Verification items for the finished model (mm, model axes). A direction names the side the tool comes from. Give positions to 0.01 mm unless a question says otherwise; leave off trailing zeros. Loops run counter-clockwise (first coordinate to the right, second up) from the corner with the lowest first, then second, coordinate; pieces in that order, holes last. Notation, with made-up numbers: (41.5, -32) - (55.5, -32) arc R15 ccw to (55.5, -20) - close; hole circle Ø5 at (48.25, 66.25). An arc over 180 degrees is marked (long way). Answer in a Markdown table with one row per item.
```python
from build123d import *

# Parameters (mm, degrees)
SKETCH_1_W           = 250
SKETCH_1_H           = 250
EXTRUDE_1_DEPTH      = 3
SKETCH_2_W           = 250
SKETCH_2_H           = 250
SKETCH_2_W_2         = 240
SKETCH_2_H_2         = 240
EXTRUDE_2_DEPTH      = 250
SKETCH_3_W           = 3
SKETCH_3_H           = 240
EXTRUDE_3_DEPTH      = 250
SKETCH_8_W           = 200
SKETCH_8_H           = 165
CUT_EXTRUDE_4_DEPTH  = 8
SKETCH_9_W           = 220
SKETCH_9_H           = 185
CUT_EXTRUDE_5_DEPTH  = 3
SKETCH_11_W          = 142
SKETCH_11_H          = 168
CUT_EXTRUDE_6_DEPTH  = 10
SKETCH_12_W          = 162
SKETCH_12_H          = 188
CUT_EXTRUDE_7_DEPTH  = 3
SKETCH_16_W          = 26
SKETCH_16_H          = 18
CUT_EXTRUDE_10_DEPTH = 5
SKETCH_17_W          = 9
SKETCH_17_H          = 11
SKETCH_17_W_2        = 15
SKETCH_17_H_2        = 8
CUT_EXTRUDE_11_DEPTH = 10
SKETCH_21_W          = 28
SKETCH_21_H          = 28
CUT_EXTRUDE_14_DEPTH = 3
SKETCH_22_W          = 50
SKETCH_22_H          = 3
EXTRUDE_4_DEPTH      = 240
SKETCH_24_R          = 4
CUT_EXTRUDE_15_DEPTH = 10
SKETCH_25_W          = 210
SKETCH_25_H          = 132
CUT_EXTRUDE_16_DEPTH = 10
SKETCH_26_R          = 1.25
CUT_EXTRUDE_17_DEPTH = 10
SKETCH_27_R          = 5
CUT_EXTRUDE_18_DEPTH = 10
SKETCH_29_W          = 35
SKETCH_29_H          = 70
CUT_EXTRUDE_19_DEPTH = 10
SKETCH_30_R          = 1.25
CUT_EXTRUDE_20_DEPTH = 3
SKETCH_31_W          = 3
SKETCH_31_H          = 15
EXTRUDE_5_DEPTH      = 3
SKETCH_32_W          = 3
SKETCH_32_H          = 15
EXTRUDE_6_DEPTH      = 3
SKETCH_33_R          = 1.25
CUT_EXTRUDE_21_DEPTH = 7
FILLET_1_R           = 3


with BuildPart() as part:
    # Эскиз1 → Бобышка-Вытянуть1 (new body)
    with BuildSketch(Plane(origin=(0, 0, 0), x_dir=(1, 0, 0), z_dir=(0, 1, 0))):
        Rectangle(SKETCH_1_W, SKETCH_1_H)
    extrude(amount=EXTRUDE_1_DEPTH)

    # Эскиз2 → Бобышка-Вытянуть2 (add)
    with BuildSketch(Plane(origin=(0, 3, 0), x_dir=(1, 0, 0), z_dir=(0, 1, 0))):
        Rectangle(SKETCH_2_W, SKETCH_2_H)
        Rectangle(SKETCH_2_W_2, SKETCH_2_H_2, mode=Mode.SUBTRACT)
    extrude(amount=EXTRUDE_2_DEPTH)

    # Эскиз3 → Бобышка-Вытянуть3 (add)
    with BuildSketch(Plane(origin=(0, 3, 0), x_dir=(1, 0, 0), z_dir=(0, 1, 0))):
        with Locations((-68.5, 0)):
            Rectangle(SKETCH_3_W, SKETCH_3_H)
    extrude(amount=EXTRUDE_3_DEPTH)

    # Эскиз8 → Вырез-Вытянуть4 (cut)
    with BuildSketch(Plane(origin=(125, 0, 0), x_dir=(0, 0, -1), z_dir=(1, 0, 0))):
        with Locations((0, 155.5)):
            Rectangle(SKETCH_8_W, SKETCH_8_H)
    extrude(amount=-CUT_EXTRUDE_4_DEPTH, mode=Mode.SUBTRACT)

    # Эскиз9 → Вырез-Вытянуть5 (cut)
    with BuildSketch(Plane.ZY.offset(-120)):
        with Locations((0, 155.5)):
            Rectangle(SKETCH_9_W, SKETCH_9_H)
    extrude(amount=-CUT_EXTRUDE_5_DEPTH, mode=Mode.SUBTRACT)

    # Эскиз11 → Вырез-Вытянуть6 (cut)
    with BuildSketch(Plane.XY.offset(125)):
        with Locations((29, 154)):
            Rectangle(SKETCH_11_W, SKETCH_11_H)
    extrude(amount=-CUT_EXTRUDE_6_DEPTH, mode=Mode.SUBTRACT)

    # Эскиз12 → Вырез-Вытянуть7 (cut)
    with BuildSketch(Plane(origin=(0, 0, 120), x_dir=(-1, 0, 0), z_dir=(0, 0, -1))):
        with Locations((-29, 154)):
            Rectangle(SKETCH_12_W, SKETCH_12_H)
    extrude(amount=-CUT_EXTRUDE_7_DEPTH, mode=Mode.SUBTRACT)

    # Эскиз16 → Вырез-Вытянуть10 (cut)
    with BuildSketch(Plane.XY.offset(125)):
        with Locations((-95, 128)):
            Rectangle(SKETCH_16_W, SKETCH_16_H)
    extrude(amount=-CUT_EXTRUDE_10_DEPTH, mode=Mode.SUBTRACT)

    # Эскиз17 → Вырез-Вытянуть11 (cut)
    with BuildSketch(Plane.ZY.offset(125)):
        with Locations((105.5, 80.5)):
            Rectangle(SKETCH_17_W, SKETCH_17_H)
        with Locations((73.5, 79)):
            Rectangle(SKETCH_17_W_2, SKETCH_17_H_2)
    extrude(amount=-CUT_EXTRUDE_11_DEPTH, mode=Mode.SUBTRACT)

    # Эскиз21 → Вырез-Вытянуть14 (cut)
    with BuildSketch(Plane(origin=(0, 0, 120), x_dir=(-1, 0, 0), z_dir=(0, 0, -1))):
        with Locations((95, 128)):
            Rectangle(SKETCH_21_W, SKETCH_21_H)
    extrude(amount=-CUT_EXTRUDE_14_DEPTH, mode=Mode.SUBTRACT)

    # Эскиз22 → Бобышка-Вытянуть4 (add)
    with BuildSketch(Plane.XY.offset(-120)):
        with Locations((-95, 71.5)):
            Rectangle(SKETCH_22_W, SKETCH_22_H)
    extrude(amount=EXTRUDE_4_DEPTH)

    # Эскиз24 → Вырез-Вытянуть15 (cut)
    with BuildSketch(Plane(origin=(-67, 0, 0), x_dir=(0, 0, -1), z_dir=(1, 0, 0))):
        with Locations((110, 65)):
            Circle(SKETCH_24_R)
    extrude(amount=-CUT_EXTRUDE_15_DEPTH, mode=Mode.SUBTRACT)

    # Эскиз25 → Вырез-Вытянуть16 (cut)
    with BuildSketch(Plane.ZY.offset(125)):
        with Locations((0, 167)):
            Rectangle(SKETCH_25_W, SKETCH_25_H)
    extrude(amount=-CUT_EXTRUDE_16_DEPTH, mode=Mode.SUBTRACT)

    # Эскиз26 → Вырез-Вытянуть17 (cut)
    with BuildSketch(Plane.ZY.offset(125)):
        with Locations((-110, 238)):
            Circle(SKETCH_26_R)
        with Locations((110, 238)):
            Circle(SKETCH_26_R)
        with Locations((110, 96)):
            Circle(SKETCH_26_R)
        with Locations((-110, 96)):
            Circle(SKETCH_26_R)
    extrude(amount=-CUT_EXTRUDE_17_DEPTH, mode=Mode.SUBTRACT)

    # Эскиз27 → Вырез-Вытянуть18 (cut)
    with BuildSketch(Plane(origin=(0, 73, 0), x_dir=(1, 0, 0), z_dir=(0, 1, 0))):
        with Locations(Location((-95, 10, 0), (0, 0, 270))):
            Circle(SKETCH_27_R)
    extrude(amount=-CUT_EXTRUDE_18_DEPTH, mode=Mode.SUBTRACT)

    # Эскиз29 → Вырез-Вытянуть19 (cut)
    with BuildSketch(Plane(origin=(0, 73, 0), x_dir=(1, 0, 0), z_dir=(0, 1, 0))):
        with Locations((-95, 65)):
            Rectangle(SKETCH_29_W, SKETCH_29_H)
    extrude(amount=-CUT_EXTRUDE_19_DEPTH, mode=Mode.SUBTRACT)

    # Эскиз30 → Вырез-Вытянуть20 (cut)
    with BuildSketch(Plane(origin=(0, 73, 0), x_dir=(1, 0, 0), z_dir=(0, 1, 0))):
        with Locations(Location((-75, 105, 0), (0, 0, 270))):
            Circle(SKETCH_30_R)
        with Locations(Location((-115, 105, 0), (0, 0, 270))):
            Circle(SKETCH_30_R)
        with Locations(Location((-115, 25, 0), (0, 0, 270))):
            Circle(SKETCH_30_R)
        with Locations(Location((-75, 25, 0), (0, 0, 270))):
            Circle(SKETCH_30_R)
    extrude(amount=-CUT_EXTRUDE_20_DEPTH, mode=Mode.SUBTRACT)

    # Эскиз31 → Бобышка-Вытянуть5 (add)
    with BuildSketch(Plane.XY.offset(-120)):
        with Locations((118.5, 245.5)):
            Rectangle(SKETCH_31_W, SKETCH_31_H)
        with Locations((-118.5, 245.5)):
            Rectangle(SKETCH_31_W, SKETCH_31_H)
    extrude(amount=EXTRUDE_5_DEPTH)

    # Эскиз32 → Бобышка-Вытянуть6 (add)
    with BuildSketch(Plane(origin=(0, 0, 120), x_dir=(-1, 0, 0), z_dir=(0, 0, -1))):
        with Locations((-118.5, 245.5)):
            Rectangle(SKETCH_32_W, SKETCH_32_H)
        with Locations((118.5, 245.5)):
            Rectangle(SKETCH_32_W, SKETCH_32_H)
    extrude(amount=EXTRUDE_6_DEPTH)

    # Эскиз33 → Вырез-Вытянуть21 (cut)
    with BuildSketch(Plane(origin=(0, 253, 0), x_dir=(1, 0, 0), z_dir=(0, 1, 0))):
        with Locations(Location((-121, -121, 0), (0, 0, 270))):
            Circle(SKETCH_33_R)
        with Locations(Location((-121, 121, 0), (0, 0, 270))):
            Circle(SKETCH_33_R)
        with Locations(Location((121, 121, 0), (0, 0, 270))):
            Circle(SKETCH_33_R)
        with Locations(Location((121, -121, 0), (0, 0, 270))):
            Circle(SKETCH_33_R)
    extrude(amount=-CUT_EXTRUDE_21_DEPTH, mode=Mode.SUBTRACT)

    # Скругление1
    fillet_1_edges = [part.edges().sort_by_distance(p)[0] for p in [
        (117, 245.5, -117),
        (-117, 245.5, -117),
        (117, 245.5, 117),
        (-117, 245.5, 117),
    ]]
    fillet(fillet_1_edges, radius=FILLET_1_R - 0.0001)  # a hair under: the kernel refuses the full size


solid = part.part
```
Q1. Draft check along X on faces 1 (the face through (-30, 69, 125)), 2 (the face through (-125, 97, 2)), 3 (the face through (-95, 73, 25)). Enter one of: +X half, -X half, draft (parallel to the pull), parting line (faces both ways), or undercut.
Completed:
| item | result |
|---|---|
| face 1 | draft |
| face 2 | -X half |
| face 3 | undercut |
Q2. Thickness scan on line 1 (X direction, y = 71.15, z = -10); line 2 (X direction, y = 249, z = 121); line 3 (Y direction, x = -109.5, z = 62). Record the ranges inside material, lowest first.
Completed:
| item | result |
|---|---|
| line 1 | -125 to -100, -90 to -67, 123 to 125 |
| line 2 | -125 to -122.25, -119.75 to 119.75, 122.25 to 125 |
| line 3 | 0 to 3, 70 to 73 |
Q3. Sectioned sample at C-C (z = -10). Give the number of separate pieces and of enclosed holes in the cut face, and give its area (4 significant figures).
Completed:
| item | result |
|---|---|
| separate pieces | 3 |
| enclosed holes | 0 |
| area | 2,575 mm^2 |
Q4. Tool access check on faces 4 (the face through (-70, 36, 2)), 5 (the face through (-99.88, 71.52, -11.08)), 6 (the face through (-56, 253, -121)). Record the directions out of +Z, -Z, +X, -X, +Y, -Y that give a thin tool (end or side, any length) a straight path to the whole face; none if there is none.
Completed:
| item | result |
|---|---|
| face 4 | none |
| face 5 | +Y |
| face 6 | +Z, -Z, +X, -X, +Y |
Q5. Go/stop test with flat-tipped pins: P1, Ø1, axis at y = 124, z = 89, coming from the -X side; P2, Ø10, axis at x = -37.5, z = -57, coming from the +Y side. Record where each tip stops, or that it passes through.
Completed:
| item | result |
|---|---|
| P1 | x = -70 |
| P2 | y = 3 |
Q6. Sectioned sample at A-A (z = 91.5). Record the cut outline in (x, y).
Completed:
| item | result |
|---|---|
| outline | (-125, 0) - (125, 0) - (125, 73) - (123, 73) - (123, 63) - (120, 63) - (120, 3) - (-67, 3) - (-67, 253) - (-70, 253) - (-70, 73) - (-120, 73) - (-120, 101) - (-125, 101) - close; (-125, 233) - (-120, 233) - (-120, 253) - (-125, 253) - close; (120, 248) - (123, 248) - (123, 238) - (125, 238) - (125, 253) - (120, 253) - close; hole (-120, 3) - (-70, 3) - (-70, 70) - (-120, 70) - close |
